```python
from build123d import *

# Parameters (mm, degrees)
SKETCH026_R     = 50
PAD008_DEPTH    = 2
SKETCH027_R     = 45.75
SKETCH027_R_2   = 43.75
PAD009_DEPTH    = 4
POCKET012_DEPTH = 4
PAD010_DEPTH    = 5


with BuildPart() as part:
    # Sketch026 → Pad008 (new body)
    with BuildSketch(Plane.XY.offset(-52)):
        Circle(SKETCH026_R)
    extrude(amount=PAD008_DEPTH)

    # Sketch027 (on Face3 of Pad008) → Pad009 (join)
    with BuildSketch(Plane.XY.offset(-50)):
        Circle(SKETCH027_R)
        Circle(SKETCH027_R_2, mode=Mode.SUBTRACT)
    extrude(amount=PAD009_DEPTH)

    # Sketch029 (on Face5 of Pad009) → Pocket012 (cut)
    with BuildSketch(Plane.XY.offset(-46)):
        Polygon((46.84259, 0), (46.84259, 5), (41.84259, 5), (41.84259, 0), (41.84259, -5), (46.84259, -5), align=None)
    extrude(amount=-POCKET012_DEPTH, mode=Mode.SUBTRACT)

    # Sketch030 → Pad010 (join, symmetric)
    with BuildSketch(Plane.XZ):
        Polygon((28.213385, -50), (28.213385, -29.455622), (-6.976082, 5.043167), (-11.961835, 5.043167), (-11.961835, -50), align=None)
        Polygon((-7.961835, 0.407958), (24.213385, -31.135746), (24.213385, -46), (-7.961835, -46), align=None, mode=Mode.SUBTRACT)
    extrude(amount=PAD010_DEPTH, both=True)


solid = part.part
```
Geometry: final body of the model. Coordinates: model frame, mm. A direction names the side the tool comes from. Round coordinates to 2 decimals unless told otherwise and drop trailing zeros. Write each loop counter-clockwise with the first axis right and the second up, starting at its lowest first coordinate (ties: lowest second). Pieces come first, ordered by that corner, then holes. Notation, with made-up numbers: (-22, -33.5) -> (5, -33.5) arc R10 ccw to (5, -19.5) -> close; hole circle Ø10 at (82, -34). An arc over 180 degrees is marked (long way). Use CSV: the item, a comma, the result in double quotes. Start each with the question number.
Q1. Section B-B (y = 0). Return loops of the section in (x, z), plus the area to 3 significant figures.
Q2. Pull-direction query (Y, two-part tool) for faces 1 (the face through (0, -44, -46)), 2 (the face through (-1, 12, -50)), 3 (the face through (47.69, 15.02, -51.01)); classes: pulls with the +Y half, pulls with the -Y half, needs draft (parallel to the pull), parting line crosses it, or undercut.
Q3. Reachability of faces 4 (the face through (28.213, 0, -40)), 5 (the face through (24.213, 0, -38)), 6 (the face through (-1, 1, -52)), 7 (the face through (10, 5, -16)), 8 (the face through (10.865, -0.07, -12.448)) from +Z, -Z, +X, -X, +Y, -Y: full face, straight path, thin tool, end or side. Return the list, or none.
Q4. Section A-A (z = -41). Return loops of the section in (x, y), plus the area to 3 significant figures.
Q5. First-contact query: pin 1 Ø11 at (y, z) = (-2, -36.5) entering from +X; pin 2 Ø3 at (y, z) = (1, -37.5) entering from -X; pin 3 Ø4 at (x, y) = (-11.5, -24) entering from +Z. Flat tips, straight axial feed; report the tip coordinate or a pass-through.
Q6. Section C-C (x = 0). Return loops of the section in (y, z).
Q7. Section D-D (x = 36.5). Return loops of the section in (y, z).
Q8. Line query: L1, parallel to Y at x = 0, z = -48.65; L2, parallel to X at y = 0, z = -47.7; L3, parallel to Z at x = -10.5, y = -14.5. Output: solid intervals per line, ascending.
Result sheet:
1,outline,"(-50, -52) -> (50, -52) -> (50, -50) -> (28.21, -50) -> (28.21, -29.46) -> (-6.98, 5.04) -> (-11.96, 5.04) -> (-11.96, -50) -> (-43.75, -50) -> (-43.75, -46) -> (-45.75, -46) -> (-45.75, -50) -> (-50, -50) -> close; hole (-7.96, -46) -> (24.21, -46) -> (24.21, -31.14) -> (-7.96, 0.41) -> close"
1,area,"827 mm²"
2,face 1,"needs draft"
2,face 2,"undercut"
2,face 3,"parting line crosses it"
3,face 4,"+Z, +X"
3,face 5,"+Y, -Y"
3,face 6,"-Z, +X, -X, +Y, -Y"
3,face 7,"+Z"
3,face 8,"+Z, +X, +Y, -Y"
4,outline,"(-11.96, -5) -> (-7.96, -5) -> (-7.96, 5) -> (-11.96, 5) -> close; (24.21, -5) -> (28.21, -5) -> (28.21, 5) -> (24.21, 5) -> close"
4,area,"80.0 mm²"
5,pin 1,"x = 28.21"
5,pin 2,"x = -11.96"
5,pin 3,"z = -50"
6,outline,"(-50, -52) -> (50, -52) -> (50, -50) -> (45.75, -50) -> (45.75, -46) -> (43.75, -46) -> (43.75, -50) -> (5, -50) -> (5, -46) -> (-5, -46) -> (-5, -50) -> (-43.75, -50) -> (-43.75, -46) -> (-45.75, -46) -> (-45.75, -50) -> (-50, -50) -> close; (-5, -7.4) -> (5, -7.4) -> (5, -1.8) -> (-5, -1.8) -> close"
7,outline,"(-34.17, -52) -> (34.17, -52) -> (34.17, -50) -> (27.58, -50) -> (27.58, -46) -> (24.12, -46) -> (24.12, -50) -> (-24.12, -50) -> (-24.12, -46) -> (-27.58, -46) -> (-27.58, -50) -> (-34.17, -50) -> close"
8,L1,"-45.75 to -43.75, -5 to 5, 43.75 to 45.75"
8,L2,"-45.75 to -43.75, -11.96 to 28.21"
8,L3,"-52 to -50"
